Design review of the part built by this model. Coordinates are the model's own, in mm. Coordinates: 2 decimals unless noted, no trailing zeros. Loops run counter-clockwise (first coordinate to the right, second up) from the corner with the lowest first, then second, coordinate; pieces in that order, holes last. Notation, with made-up numbers: (28.25, 53.5) -> (57.25, 53.5) arc R23 cw to (57.25, 64.5) -> close; hole circle Ø9 at (-27, 32.5). An arc over 180 degrees is marked (long way). Answer as a JSON object with one key per item and string values.
Autodesk Fusion 360 part; units mm, degrees
sketch "草图1" plane through (0, 0, 0) normal (0, 1, 0) x (1, 0, 0)
  circle A0 centre (0, 0) radius 40.6099
  arc A1 (22.6638, -30.0143) -> (36.1396, 10.4131) centre (0, 0) ccw
  arc A2 (35.5488, 12.2796) -> (1.2643, 37.5886) centre (0, 0) ccw
  arc A3 (-21.5418, -30.8295) -> (21.0712, -31.153) centre (0, 0) ccw
  arc A4 (-0.6935, 37.6035) -> (-35.3582, 12.8179) centre (0, 0) ccw
  arc A5 (-35.9774, 10.9606) -> (-23.1169, -29.6667) centre (0, 0) ccw
  line L0 (-9.022, 12.618) -> (-35.3582, 12.8179)
  line L1 (-10.0195, 9.6255) -> (-29.3159, 9.772)
  line L2 (0.2346, 30.9008) -> (-5.8677, 12.5941)
  line L3 (-0.6935, 37.6035) -> (-9.022, 12.618)
  line L4 (0.2346, 30.9008) -> (6.0582, 12.5035)
  line L5 (35.5488, 12.2796) -> (9.2125, 12.4796)
  line L6 (6.0582, 12.5035) -> (-5.8677, 12.5941)
  line L7 (1.2643, 37.5886) -> (9.2125, 12.4796)
  line L8 (29.4609, 9.3258) -> (10.1644, 9.4723)
  line L9 (7.0102, 9.4962) -> (-6.8652, 9.6015)
  line L10 (13.7636, -1.8979) -> (29.4609, 9.3258)
  line L11 (14.7156, -4.9052) -> (36.1396, 10.4131)
  line L12 (7.0102, 9.4962) -> (11.1977, -3.7326)
  line L13 (12.1496, -6.7399) -> (17.9733, -25.1372)
  line L14 (10.1644, 9.4723) -> (13.7636, -1.8979)
  line L15 (14.7156, -4.9052) -> (22.6638, -30.0143)
  line L16 (17.9733, -25.1372) -> (2.4482, -13.6765)
  line L17 (21.0712, -31.153) -> (-0.1178, -15.5112)
  line L18 (-18.3528, -24.8614) -> (-2.6556, -13.6377)
  line L19 (-0.0896, -11.8031) -> (11.1977, -3.7326)
  line L20 (-21.5418, -30.8295) -> (-0.1178, -15.5112)
  line L21 (2.4482, -13.6765) -> (12.1496, -6.7399)
  line L22 (-6.8652, 9.6015) -> (-11.2531, -3.5621)
  line L23 (-12.2506, -6.5546) -> (-18.3528, -24.8614)
  line L24 (-2.6556, -13.6377) -> (-12.2506, -6.5546)
  line L25 (-14.7884, -4.6812) -> (-35.9774, 10.9606)
  line L26 (-0.0896, -11.8031) -> (-11.2531, -3.5621)
  line L27 (-13.7909, -1.6887) -> (-29.3159, 9.772)
  line L28 (-10.0195, 9.6255) -> (-13.7909, -1.6887)
  line L29 (-14.7884, -4.6812) -> (-23.1169, -29.6667)
extrude "拉伸1" add sketch "草图1" along normal blind 5 makes body 1
sketch "草图2" plane through (0, 0, 0) normal (0, 1, 0) x (1, 0, 0)
  circle A0 centre (58.5356, 21.3067) radius 4
  circle A1 centre (58.5356, 21.3067) radius 2.5
  dimension "d6" = 8
  dimension "d7" = 5
extrude "拉伸2" add sketch "草图2" along normal blind 5 separate body makes body 2
move_body "移动1" bodies 2 to x (1, 0, 0) y (0, 1, 0) z (0, 0, 1) at (-58.3, 0, -22.5)
combine "合并1" operation add target body 1 tool bodies 2
1) Add section C-C, the plane z = 34. Give the boundary of the cut face in (x, y).
Completed:
{"outline": "(-22.21, 0) -> (-16.08, 0) -> (-16.08, 5) -> (-22.21, 5) -> close; (16.08, 0) -> (22.21, 0) -> (22.21, 5) -> (16.08, 5) -> close"}
2) Add section A-A, the plane z = -6.5. Give the boundary of the cut face in (x, y), and give its area (3 significant figures).
Completed:
{"outline": "(-40.09, 0) -> (-37.04, 0) -> (-37.04, 5) -> (-40.09, 5) -> close; (-29.93, 0) -> (-24.88, 0) -> (-24.88, 5) -> (-29.93, 5) -> close; (-11.06, 0) -> (-7.9, 0) -> (-7.9, 5) -> (-11.06, 5) -> close; (7.96, 0) -> (11.11, 0) -> (11.11, 5) -> (7.96, 5) -> close; (25.51, 0) -> (30.67, 0) -> (30.67, 5) -> (25.51, 5) -> close; (37.04, 0) -> (40.09, 0) -> (40.09, 5) -> (37.04, 5) -> close", "area": "113 mm²"}
3) Add section D-D, the plane x = 20. Give the boundary of the cut face in (y, z), and give its area (3 significant figures).
Completed:
{"outline": "(0, -35.34) -> (5, -35.34) -> (5, -31.85) -> (0, -31.85) -> close; (0, -12.4) -> (5, -12.4) -> (5, -9.4) -> (0, -9.4) -> close; (0, -2.56) -> (5, -2.56) -> (5, 1.13) -> (0, 1.13) -> close; (0, 21.6) -> (5, 21.6) -> (5, 30.36) -> (0, 30.36) -> close; (0, 31.85) -> (5, 31.85) -> (5, 35.34) -> (0, 35.34) -> close", "area": "112 mm²"}
4) Wall thickness on probe 1 along X at (y, z) = (0.7, 0.5); probe 2 along Z at (x, y) = (28, 1.65); probe 3 along Z at (x, y) = (26.5, 0.7): over which ranges is each line inside the solid? List them lowest first.
Completed:
{"probe 1": "-40.61 to -37.61, -20.45 to -15.4, -13.39 to -10.23, 10.17 to 13.32, 15.72 to 20.88, 37.61 to 40.61", "probe 2": "-29.41 to -25.11, -12.34 to -9.34, -8.28 to -4.59, 25.11 to 29.41", "probe 3": "-30.77 to -26.69, -12.35 to -9.35, -7.21 to -3.52, 26.69 to 30.77"}
5) Add section B-B, the plane x = -31. Give the boundary of the cut face in (y, z).
Completed:
{"outline": "(0, -26.23) -> (5, -26.23) -> (5, -21.3) -> (0, -21.3) -> close; (0, -12.78) -> (5, -12.78) -> (5, -7.29) -> (0, -7.29) -> close; (0, 21.3) -> (5, 21.3) -> (5, 26.23) -> (0, 26.23) -> close"}
6) Clearance check with flat-ended pins moving along their axes: pin 1 Ø2 at (x, z) = (13.5, -14.5) entering from +Y; pin 2 Ø1 at (x, z) = (-10.5, 4) entering from +Y; pin 3 Ø3 at (x, y) = (-10, 0.5) entering from -Z. State where each tip first meets the part, or that it passes through.
Completed:
{"pin 1": "through", "pin 2": "y = 5", "pin 3": "z = -39.71"}
